Could you check a few things on this model? Use its own coordinates, in mm. Face numbers are marked on the shaded views. A direction names the side the tool comes from. Round coordinates to 2 decimals unless told otherwise and drop trailing zeros. Order: outer loops, then holes, each group sorted by start corner. A loop starts at its lowest first (then second) coordinate and runs counter-clockwise, first axis right, second up. Notation, with made-up numbers: (-9.5, 63) -> (3.5, 63) arc R22 ccw to (3.5, 82) -> close; hole circle Ø11 at (40, 14.5). An arc over 180 degrees is marked (long way). Put each result on its own line as item: value. Start each with the question number.
Autodesk Inventor part; units mm, degrees
ref_plane "YZ Plane" through (0, 0, 0) normal (1, 0, 0) x (0, 1, 0)
ref_plane "XZ Plane" through (0, 0, 0) normal (0, 1, 0) x (-1, 0, 0)
ref_plane "XY Plane" through (0, 0, 0) normal (0, 0, 1) x (1, 0, 0)
sketch "Sketch1" plane through (0, 0, 0) normal (0, 0, 1) x (1, 0, 0)
  line L0 (-3.5, 3.5) -> (3.5, 3.5)
  line L1 (3.5, 3.5) -> (3.5, -3.5)
  line L2 (3.5, -3.5) -> (-3.5, -3.5)
  line L3 (-3.5, -3.5) -> (-3.5, 3.5)
  line L4 (-4.5, 4.5) -> (4.5, 4.5)
  line L5 (4.5, 4.5) -> (4.5, -4.5)
  line L6 (4.5, -4.5) -> (-4.5, -4.5)
  line L7 (-4.5, -4.5) -> (-4.5, 4.5)
  line L8 (-1, -3.5) -> (-1, -4.5)
  line L9 (1, -3.5) -> (1, -4.5)
  point P0 (0, 0)
  point P1 (0, 3.5)
  point P2 (-3.5, 0)
  point P3 (-4.5, 0)
  point P4 (0, 4.5)
  dimension "d0" = 1
  dimension "d1" = 1
  dimension "d2" = 7
  dimension "d3" = 7
  dimension "d4" = 2
  dimension "d5" = 1
extrude "Extrusion1" add sketch "Sketch1" along normal blind 3.5 contours L3 L2 L8 L6 L7 L4 L5 L9 L1 L0
fillet "Fillet1" radius 1 4 edges at (4.5, 4.5, 1.75) (-4.5, 4.5, 1.75) (-4.5, -4.5, 1.75) (4.5, -4.5, 1.75)
equation "\"d1\" = d0"
properties part number "cable_clip_rev1"
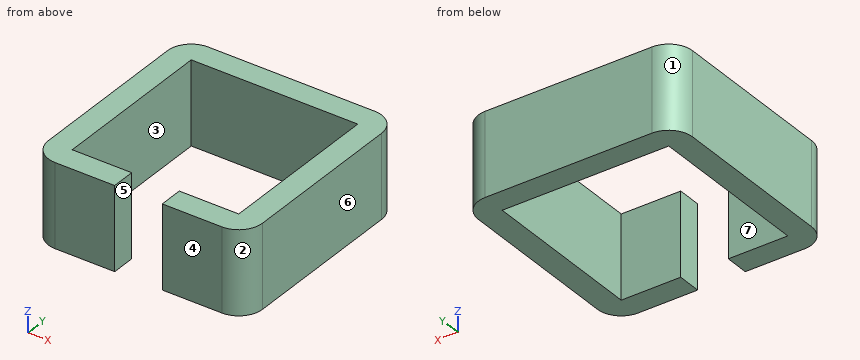
1. I need wall thicknesses on L1, parallel to Y at x = -2.5, z = 0.35; L2, parallel to Y at x = 0, z = 2.65. Which ranges of each line are inside material? Lowest first, please.
2. If we section it at C-C, the plane z = 0.35: Please give me the cut outline in (x, y).
3. If we section it at D-D, the plane x = 4: Please give me the cut outline in (y, z).
4. Thinking about a two-plate mould opening in X: for the marked faces 1, 2, 3 and 4, which applies, +X half, -X half, draft (parallel to the pull), parting line (faces both ways), or undercut?
5. If we section it at A-A, the plane y = 2.75: Please give me the cut outline in (x, z), then the cut area to 3 significant figures.
6. For pin 1 Ø0.5 at (y, z) = (-4, 2) entering from -X; pin 2 Ø0.8 at (y, z) = (-4, 2.5) entering from +X (3 decimals), each with a flat end and sliding along its axis, tell me the tip position at first contact or that it passes through.
7. Which directions (+Z, -Z, +X, -X, +Y, -Y) give clear straight access to the entire face, cutting with the end or side of a thin tool? Please do the marked faces 5, 6 and 7.
Results below:
1. L1: -4.5 to -3.5, 3.5 to 4.5
1. L2: 3.5 to 4.5
2. outline: (-4.5, -3.5) arc R1 ccw to (-3.5, -4.5) -> (-1, -4.5) -> (-1, -3.5) -> (-3.5, -3.5) -> (-3.5, 3.5) -> (3.5, 3.5) -> (3.5, -3.5) -> (1, -3.5) -> (1, -4.5) -> (3.5, -4.5) arc R1 ccw to (4.5, -3.5) -> (4.5, 3.5) arc R1 ccw to (3.5, 4.5) -> (-3.5, 4.5) arc R1 ccw to (-4.5, 3.5) -> close
3. outline: (-4.37, 0) -> (4.37, 0) -> (4.37, 3.5) -> (-4.37, 3.5) -> close
4. face 1: -X half
4. face 2: +X half
4. face 3: undercut
4. face 4: draft
5. outline: (-4.5, 0) -> (-3.5, 0) -> (-3.5, 3.5) -> (-4.5, 3.5) -> close; (3.5, 0) -> (4.5, 0) -> (4.5, 3.5) -> (3.5, 3.5) -> close
5. area: 7.00 mm2
6. pin 1: x = -4.47
6. pin 2: x = 4.495
7. face 5: +Z, -Z, -Y
7. face 6: +Z, -Z, +X, +Y, -Y
7. face 7: +Z, -Z
